Geometry check sheet. Reference: the model listing, model coordinates, mm. A direction names the side the tool comes from. Round coordinates to 2 decimals unless told otherwise and drop trailing zeros. Write each loop counter-clockwise with the first axis right and the second up, starting at its lowest first coordinate (ties: lowest second). Pieces come first, ordered by that corner, then holes. Notation, with made-up numbers: M 74,59.5 L 125,59.5 A32 cw 125,92.5 Z; hole C 87,34.5 d2. An arc over 180 degrees is marked long. Put each result on its own line as item: value. Start each with the question number.
(1) Section check D-D on y = 16. Record the cut outline in (x, z), then the cut area to 3 significant figures.
(2) Section check A-A on y = 0. Count the separate pieces of the cut face and the enclosed holes in it, then the cut area to 3 significant figures.
(3) Tool access check on faces 1 (the flat face through (2.9, 4, 56)), 2 (the flat face through (-9, 0, 3)), 3 (the flat face through (-4, -2.9, 56)). Record the directions out of +Z, -Z, +X, -X, +Y, -Y that give a thin tool (end or side, any length) a straight path to the whole face; none if there is none.
(4) Gauge pin test, flat ends, axial feed: pin 1 (1.8 mm diameter, centred on x = 4.5, z = 2, fed in from +Y); pin 2 (4 mm diameter, centred on x = 0, y = 0, fed in from -Z); pin 3 (3 mm diameter, centred on x = -6, z = 2.5, fed in from -Y). Record the tip position at first contact, or that the pin passes through.
(5) Section check B-B on x = 22.5. Record the cut outline in (y, z).
(6) Material ranges on probe 1 along Y at (x, z) = (-10.5, 7); probe 2 along Z at (x, y) = (-5, -4); probe 3 along Z at (x, y) = (15, 20.5), recorded low to high.
(7) Mould release check, pull along X, two halves, no side actions. Record for faces 4 (the flat face through (-4, 2.9, 56)), 5 (the flat face through (-2, -5, 3)), 6 (the cylindrical face through (27.136, -8.546, 4.141)): pulls with the +X half, pulls with the -X half, needs draft (parallel to the pull), parting line crosses it, or undercut.
(8) Section check C-C on z = 31. Record the cut outline in (x, y).
Autodesk Inventor part; units mm, degrees
ref_plane "YZ Plane" through (0, 0, 0) normal (1, 0, 0) x (0, 1, 0)
ref_plane "XZ Plane" through (0, 0, 0) normal (0, 1, 0) x (-1, 0, 0)
ref_plane "XY Plane" through (0, 0, 0) normal (0, 0, 1) x (1, 0, 0)
sketch "Sketch1" plane through (0, 0, 0) normal (0, 0, 1) x (1, 0, 0)
  circle A0 centre (0, 0) radius 28.45
  dimension "d0" = 56.9
extrude "Extrusion1" add sketch "Sketch1" along normal blind 8.4
sketch "Sketch2" plane through (0, 0, 8.4) normal (0, 0, 1) x (1, 0, 0)
  line L0 (0, 0) -> (23.85, 0)
  line L1 (0, 0) -> (11.925, 20.6547)
  line L2 (0, 0) -> (23.85, 0) construction
  line L3 (0, 0) -> (-11.925, 20.6547)
  line L4 (0, 0) -> (23.85, 0) construction
  line L5 (0, 0) -> (-23.85, 0)
  line L6 (0, 0) -> (23.85, 0) construction
  line L7 (0, 0) -> (11.925, -20.6547)
  line L8 (0, 0) -> (23.85, 0) construction
  line L9 (0, 0) -> (-11.925, -20.6547)
  line L10 (0, 0) -> (23.85, 0) construction
  circle A0 centre (23.85, 0) radius 2.5
  circle A1 centre (11.925, 20.6547) radius 2.5
  circle A2 centre (11.925, -20.6547) radius 2.5
  circle A3 centre (-11.925, -20.6547) radius 2.5
  circle A4 centre (-23.85, 0) radius 2.5
  circle A5 centre (-11.925, 20.6547) radius 2.5
  dimension "d3" = 23.85
  dimension "d4" = 23.85
  dimension "d5" = 60
  dimension "d6" = 23.85
  dimension "d7" = 120
  dimension "d8" = 23.85
  dimension "d9" = 180
  dimension "d10" = 23.85
  dimension "d11" = 60
  dimension "d12" = 23.85
  dimension "d13" = 120
  dimension "d14" = 5
  dimension "d15" = 5
  dimension "d16" = 5
  dimension "d17" = 5
  dimension "d18" = 5
  dimension "d19" = 5
extrude "Extrusion2" cut sketch "Sketch2" against normal blind 8.4
sketch "Sketch3" plane through (0, 0, 8.4) normal (0, 0, 1) x (1, 0, 0)
  circle A0 centre (0, 0) radius 9.5
  dimension "d22" = 19
extrude "Extrusion3" add sketch "Sketch3" along normal blind 27
sketch "Sketch4" plane through (0, 0, 35.4) normal (0, 0, 1) x (1, 0, 0)
  circle A0 centre (0, 0) radius 8
  dimension "d25" = 16
extrude "Extrusion4" add sketch "Sketch4" along normal blind 15.5
sketch "Sketch6" plane through (0, 0, 0) normal (0, 0, -1) x (-1, 0, 0)
  line L0 (0, 0) -> (0, 9)
  line L1 (0, 9) -> (2, 9)
  line L2 (2, 9) -> (2, 2)
  line L3 (2, 2) -> (9, 2)
  line L4 (9, 2) -> (9, -2)
  line L5 (9, -2) -> (2, -2)
  line L6 (2, -2) -> (2, -9)
  line L7 (2, -9) -> (-2, -9)
  line L8 (-2, -9) -> (-2, -2)
  line L9 (-2, -2) -> (-9, -2)
  line L10 (-9, -2) -> (-9, 2)
  line L11 (-9, 2) -> (-2, 2)
  line L12 (-2, 2) -> (-2, 9)
  line L13 (-2, 9) -> (0, 9)
  dimension "d120" = 9
  dimension "d121" = 2
  dimension "d122" = 7
  dimension "d124" = 7
  dimension "d125" = 4
  dimension "d126" = 7
  dimension "d127" = 7
  dimension "d128" = 4
  dimension "d129" = 7
  dimension "d130" = 7
  dimension "d131" = 4
  dimension "d132" = 7
  dimension "d133" = 7
extrude "Extrusion6" cut sketch "Sketch6" against normal blind 6
sketch "Sketch7" plane through (0, 0, 6) normal (0, 0, -1) x (-1, 0, 0)
  circle A0 centre (0, 0) radius 1.5
  dimension "d91" = 3
extrude "Extrusion7" cut sketch "Sketch7" against normal blind 5
thread "Thread3"
sketch "Sketch12" plane through (0, 0, 50.9) normal (0, 0, 1) x (1, 0, 0)
  line L0 (0, 0) -> (5.9, 0)
  line L1 (5.9, 0) -> (5.9, 2.9)
  line L2 (5.9, 0) -> (5.9, -2.9)
  line L3 (5.9, 2.9) -> (2.9, 2.9)
  line L4 (2.9, 2.9) -> (2.9, 5.9)
  line L5 (5.9, -2.9) -> (2.9, -2.9)
  line L6 (2.9, -2.9) -> (2.9, -5.9)
  line L7 (2.9, -5.9) -> (-2.9, -5.9)
  line L8 (-2.9, -5.9) -> (-2.9, -2.9)
  line L9 (-2.9, -2.9) -> (-5.9, -2.9)
  line L10 (-5.9, -2.9) -> (-5.9, 2.9)
  line L11 (-5.9, 2.9) -> (-2.9, 2.9)
  line L12 (-2.9, 2.9) -> (-2.9, 5.9)
  line L13 (-2.9, 5.9) -> (2.9, 5.9)
  dimension "d221" = 5.9
  dimension "d222" = 2.9
  dimension "d223" = 2.9
  dimension "d224" = 3
  dimension "d225" = 3
  dimension "d226" = 3
  dimension "d227" = 3
  dimension "d228" = 5.8
  dimension "d229" = 3
  dimension "d230" = 3
  dimension "d231" = 5.8
  dimension "d232" = 3
  dimension "d233" = 3
extrude "Extrusion11" add sketch "Sketch12" along normal blind 10
properties part number "OmniWheelAxle"
Answers follow:
1. outline: M -23.52,0 L 23.52,0 L 23.52,8.4 L -23.52,8.4 Z
1. area: 395 mm^2
2. separate pieces: 3
2. enclosed holes: 0
2. area: 1,150 mm^2
3. face 1: +Z, +X, +Y
3. face 2: -Z
3. face 3: +Z, -X, -Y
4. pin 1: stops at y = 28.22
4. pin 2: stops at z = 6
4. pin 3: stops at y = -28.09
5. outline: M -17.41,0 L -2.1,0 L -2.1,8.4 L -17.41,8.4 Z; M 2.1,0 L 17.41,0 L 17.41,8.4 L 2.1,8.4 Z
6. probe 1: y = -26.44 to -22.71, -18.6 to 18.6, 22.71 to 26.44
6. probe 2: z = 0 to 50.9
6. probe 3: z = 0 to 8.4
7. face 4: needs draft
7. face 5: undercut
7. face 6: parting line crosses it
8. outline: C 0,0 d19
